The model under review builds one solid part; all positions refer to its coordinate system, in mm. Face numbers are marked on the shaded views. A direction names the side the tool comes from. Give positions to 0.01 mm unless a question says otherwise; leave off trailing zeros. Write each loop counter-clockwise with the first axis right and the second up, starting at its lowest first coordinate (ties: lowest second). Pieces come first, ordered by that corner, then holes.
from build123d import *

# Parameters (mm, degrees)
SKETCH1_W           = 109.4
SKETCH1_H           = 109.4
SKETCH1_W_2         = 79.4
SKETCH1_H_2         = 79.4
SKETCH1_R           = 6
SKETCH1_R_2         = 1.5
BOSS_EXTRUDE1_DEPTH = 8
BOSS_EXTRUDE2_DEPTH = 109.4
FILLET1_R           = 30
SKETCH5_W           = 8
SKETCH5_H           = 149.4
BOSS_EXTRUDE3_DEPTH = 109.4
SKETCH3_W           = 8
SKETCH3_H           = 109.4
CUT_EXTRUDE4_DEPTH  = 135
SKETCH7_W           = 8
SKETCH7_H           = 40
CUT_EXTRUDE5_DEPTH  = 135
SKETCH4_R           = 2.5
CUT_EXTRUDE6_DEPTH  = 10
BOSS_EXTRUDE4_START = 7.8
BOSS_EXTRUDE4_DEPTH = 7.8


with BuildPart() as part:
    # Sketch1 → Boss-Extrude1 (new body)
    # profile 1 of 2: a face of its own
    with BuildSketch(Plane.XY):
        with Locations((-17.5, 17.5)):
            Rectangle(SKETCH1_W, SKETCH1_H)
        with Locations((-17.5, 17.5)):
            Rectangle(SKETCH1_W_2, SKETCH1_H_2, mode=Mode.SUBTRACT)
    # profile 2 of 2: a face of its own
    with BuildSketch(Plane.XY):
        with Locations((-17.5, 17.5)):
            Rectangle(SKETCH1_W_2, SKETCH1_H_2)
        with Locations((-35, 0)):
            Circle(SKETCH1_R, mode=Mode.SUBTRACT)
        Circle(SKETCH1_R, mode=Mode.SUBTRACT)
        with Locations((0, 35)):
            Circle(SKETCH1_R, mode=Mode.SUBTRACT)
        with Locations((-35, 35)):
            Circle(SKETCH1_R, mode=Mode.SUBTRACT)
        with Locations((-52.809903828, -17.809903828)):
            Circle(SKETCH1_R_2, mode=Mode.SUBTRACT)
        with Locations((-17.5, -17.5)):
            Circle(SKETCH1_R_2, mode=Mode.SUBTRACT)
        with Locations((17.5, -17.5)):
            Circle(SKETCH1_R_2, mode=Mode.SUBTRACT)
        with Locations((17.5, 17.5)):
            Circle(SKETCH1_R_2, mode=Mode.SUBTRACT)
        with Locations((-17.5, 17.5)):
            Circle(SKETCH1_R_2, mode=Mode.SUBTRACT)
        with Locations((-52.5, 17.5)):
            Circle(SKETCH1_R_2, mode=Mode.SUBTRACT)
        with Locations((17.5, 52.5)):
            Circle(SKETCH1_R_2, mode=Mode.SUBTRACT)
        with Locations((-17.5, 52.5)):
            Circle(SKETCH1_R_2, mode=Mode.SUBTRACT)
        with Locations((-52.5, 52.5)):
            Circle(SKETCH1_R_2, mode=Mode.SUBTRACT)
    extrude(amount=BOSS_EXTRUDE1_DEPTH)



with BuildPart() as body_2:
    # Sketch2 → Boss-Extrude2 (new body)
    with BuildSketch(Plane(origin=(37.2, 0, 0), x_dir=(0, 0, -1), z_dir=(1, 0, 0))):
        Polygon((-8, 72.2), (-33.651510749, 1.723053441), (-29.425328132, -7.340024429), (-32.127552961, -8.237713324), (-37.410281233, 3.091134014), (-12, 72.905307923), (-12, 112.2), (-8, 112.2), align=None)
    extrude(amount=-BOSS_EXTRUDE2_DEPTH)

    # Fillet1
    fillet1_edges = [body_2.edges().sort_by_distance(p)[0] for p in [
        (-17.5, 72.905307923, 12),
    ]]
    fillet(fillet1_edges, radius=FILLET1_R)


with BuildPart() as part_1:
    add(part.part)

    add(body_2.part)  # Boss-Extrude3 merges body 2
    # Sketch5 → Boss-Extrude3 (add)
    with BuildSketch(Plane(origin=(37.2, 0, 0), x_dir=(0, 0, -1), z_dir=(1, 0, 0))):
        with Locations((-4, 37.5)):
            Rectangle(SKETCH5_W, SKETCH5_H)
    extrude(amount=-BOSS_EXTRUDE3_DEPTH)

    # Sketch3 → Cut-Extrude4 (cut)
    with BuildSketch(Plane(origin=(37.2, 0, 0), x_dir=(0, 0, -1), z_dir=(1, 0, 0))):
        with Locations((-4, 17.5)):
            Rectangle(SKETCH3_W, SKETCH3_H)
    extrude(amount=-CUT_EXTRUDE4_DEPTH, mode=Mode.SUBTRACT)

    # Sketch7 → Cut-Extrude5 (cut)
    with BuildSketch(Plane(origin=(37.2, 0, 0), x_dir=(0, 0, -1), z_dir=(1, 0, 0))):
        with Locations((-4, 92.2)):
            Rectangle(SKETCH7_W, SKETCH7_H)
    extrude(amount=-CUT_EXTRUDE5_DEPTH, mode=Mode.SUBTRACT)

    # Sketch4 → Cut-Extrude6 (cut)
    with BuildSketch(Plane.XY.offset(12)):
        with Locations((-52.8, 94.2)):
            Circle(SKETCH4_R)
        with Locations((-32.8, 94.2)):
            Circle(SKETCH4_R)
        with Locations((-12.8, 94.2)):
            Circle(SKETCH4_R)
        with Locations((7.2, 94.2)):
            Circle(SKETCH4_R)
        with Locations((27.2, 94.2)):
            Circle(SKETCH4_R)
    extrude(amount=-CUT_EXTRUDE6_DEPTH, mode=Mode.SUBTRACT)

    # Sketch8 → Boss-Extrude4 (add)
    with BuildSketch(Plane.ZY.offset(72.2).offset(BOSS_EXTRUDE4_START)):
        with BuildLine():
            Line((12, 112.2), (8, 112.2))
            Line((8, 112.2), (8, 72.2))
            Line((8, 72.2), (33.651510749, 1.723053441))
            Line((33.651510749, 1.723053441), (29.425328132, -7.340024429))
            Line((29.425328132, -7.340024429), (32.127552961, -8.237713324))
            Line((32.127552961, -8.237713324), (37.410281233, 3.091134014))
            Line((37.410281233, 3.091134014), (13.809221376, 67.934513044))
            ThreePointArc((13.809221376, 67.934513044), (12.45576741, 72.985672014), (12, 78.195117344))
            Line((12, 78.195117344), (12, 112.2))
        make_face()
    extrude(amount=-BOSS_EXTRUDE4_DEPTH)


solid = part_1.part
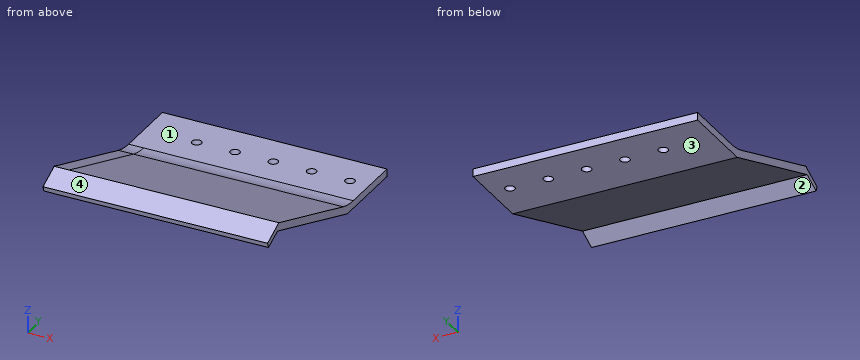
1) Consider section A-A, the plane x = -52.8. Give the boundary of the cut face in (y, z), then the cut area to 3 significant figures.
2) Consider section D-D, the plane z = 27.5. Give the boundary of the cut face in (x, y), then the cut area to 3 significant figures.
3) Consider section C-C, the plane x = 22.5. Give the boundary of the cut face in (y, z), then the cut area to 3 significant figures.
4) Tool access review of the marked faces 1 and 2: name each direction out of +Z, -Z, +X, -X, +Y, -Y from which nothing blocks a thin tool from reaching the whole face with its end or side.
5) The part is to be moulded in two halves that separate along Z. For the marked faces 3 and 4, say which applies: +Z half, -Z half, draft (parallel to the pull), parting line (faces both ways), or undercut.
6) To check wall thickness, follow probe 1 along Z at (x, y) = (14, 102.5); probe 2 along Z at (x, y) = (-8.5, 21). State the ranges of each line that lie inside material, in increasing order.
7) Consider section B-B, the plane y = 94.2. Give the boundary of the cut face in (x, z), then the cut area to 3 significant figures.
8) Insertion check: pin 1 (12 mm diameter, centred on x = -29.5, y = 23.5, fed in from -Z); pin 2 (1 mm diameter, centred on x = -24.5, y = 34, fed in from -Z); pin 3 (4 mm diameter, centred on x = 7.2, y = 94.2, fed in from +Z); pin 4 (5 mm diameter, centred on x = 1.5, y = 20.5, fed in from -Z). Each pin has a flat end and moves straight along its axis. Give the tip position at first contact, or say it passes through.
Answer block:
1. outline: (-8.24, 32.13) - (-7.34, 29.43) - (1.72, 33.65) - (72.2, 8) - (91.7, 8) - (91.7, 12) - (78.2, 12) arc R30 cw to (67.93, 13.81) - (3.09, 37.41) - close; (96.7, 8) - (112.2, 8) - (112.2, 12) - (96.7, 12) - close
1. area: 471 mm2
2. outline: (-80, 18.62) - (37.2, 18.62) - (37.2, 30.32) - (-80, 30.32) - close
2. area: 1,370 mm2
3. outline: (-8.24, 32.13) - (-7.34, 29.43) - (1.72, 33.65) - (72.2, 8) - (112.2, 8) - (112.2, 12) - (78.2, 12) arc R30 cw to (67.93, 13.81) - (3.09, 37.41) - close
3. area: 491 mm2
4. face 1: +Z, +X, -X, +Y
4. face 2: -Z, +X, -X
5. face 3: -Z half
5. face 4: +Z half
6. probe 1: z = 8 to 12
6. probe 2: z = 26.64 to 30.89
7. outline: (-80, 8) - (-55.3, 8) - (-55.3, 12) - (-80, 12) - close; (-50.3, 8) - (-35.3, 8) - (-35.3, 12) - (-50.3, 12) - close; (-30.3, 8) - (-15.3, 8) - (-15.3, 12) - (-30.3, 12) - close; (-10.3, 8) - (4.7, 8) - (4.7, 12) - (-10.3, 12) - close; (9.7, 8) - (24.7, 8) - (24.7, 12) - (9.7, 12) - close; (29.7, 8) - (37.2, 8) - (37.2, 12) - (29.7, 12) - close
7. area: 369 mm2
8. pin 1: stops at z = 23.54
8. pin 2: stops at z = 21.72
8. pin 3: passes through
8. pin 4: stops at z = 25.91
